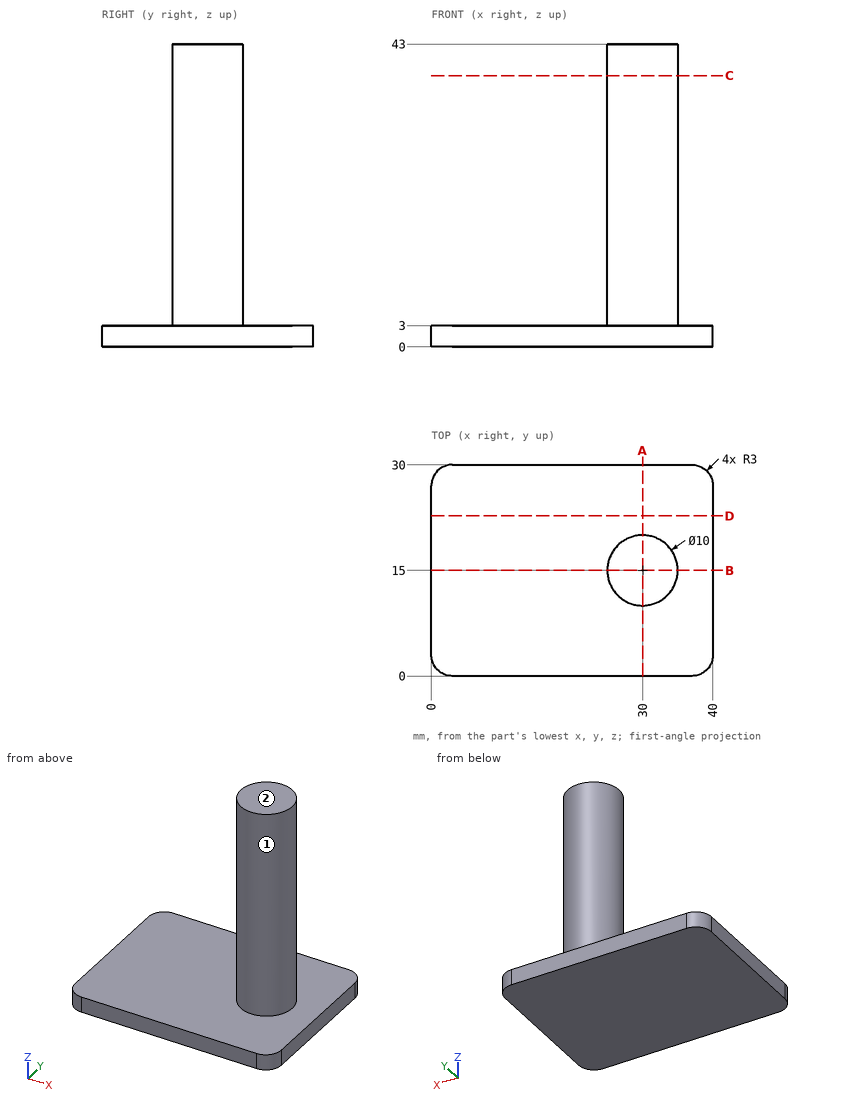
Here's the drawing with two shaded views (mm, measured from the low corner). I have some questions. A direction names the side the tool comes from. Coordinates: 2 decimals unless noted, no trailing zeros. Write each loop counter-clockwise with the first axis right and the second up, starting at its lowest first coordinate (ties: lowest second). Pieces come first, ordered by that corner, then holes. Notation, with made-up numbers: (75.25, -2) -> (134.25, -2) arc R26 cw to (134.25, 26) -> close; hole circle Ø9 at (4, -30). An arc over 180 degrees is marked (long way). One line per question, with ' | ' between items. Start each with the question number.
1. If we section it at C-C (z = 38.5): Please give me the cut outline in (x, y), and give its area (3 significant figures).
2. Will these pins go through, and if not, where does the flat tip stop? P1, Ø8, axis at y = 23, z = 13, coming from the -X side; P2, Ø2, axis at x = 30.5, z = 30.5, coming from the +Y side; P3, Ø1, axis at x = 14.5, y = 16, coming from the -Z side; P4, Ø2, axis at y = 11.5, z = 36, coming from the +X side.
3. If we section it at A-A (x = 30): Please give me the cut outline in (y, z), and give its area (3 significant figures).
4. For the marked faces 1 and 2, which set-ups out of +Z, -Z, +X, -X, +Y, -Y let a thin tool reach every point of the face, with its end or its side?
5. If we section it at D-D (y = 22.75): Please give me the cut outline in (x, z), and give its area (3 significant figures).
6. If we section it at B-B (y = 15): Please give me the cut outline in (x, z).
7. Please list where these lines run through material, in increasing order: line 1 along Z through (x, y) = (15.5, 9.25); line 2 along X through (y, z) = (17.5, 25.5); line 3 along Y through (x, z) = (29.5, 15.5).
Return value:
1) outline: circle Ø10 at (30, 15) | area: 78.5 mm²
2) P1: stops at x = 27 | P2: stops at y = 20 | P3: stops at z = 0 | P4: stops at x = 34.33
3) outline: (0, 0) -> (30, 0) -> (30, 3) -> (20, 3) -> (20, 43) -> (10, 43) -> (10, 3) -> (0, 3) -> close | area: 490 mm²
4) face 1: +Z | face 2: +Z, +X, -X, +Y, -Y
5) outline: (0, 0) -> (40, 0) -> (40, 3) -> (0, 3) -> close | area: 120 mm²
6) outline: (0, 0) -> (40, 0) -> (40, 3) -> (35, 3) -> (35, 43) -> (25, 43) -> (25, 3) -> (0, 3) -> close
7) line 1: z = 0 to 3 | line 2: x = 25.67 to 34.33 | line 3: y = 10.03 to 19.97
